Can you work these out from the drawing? Everything is in mm from the part's minimum corner. A direction names the side the tool comes from. Round coordinates to 2 decimals unless told otherwise and drop trailing zeros. Order: outer loops, then holes, each group sorted by start corner. A loop starts at its lowest first (then second) coordinate and runs counter-clockwise, first axis right, second up. Notation, with made-up numbers: (39.25, -34.5) -> (45.25, -34.5) arc R28 ccw to (45.25, 1.5) -> close; hole circle Ø8 at (67.5, -19.75). An arc over 180 degrees is marked (long way). One line per item, written item: value.
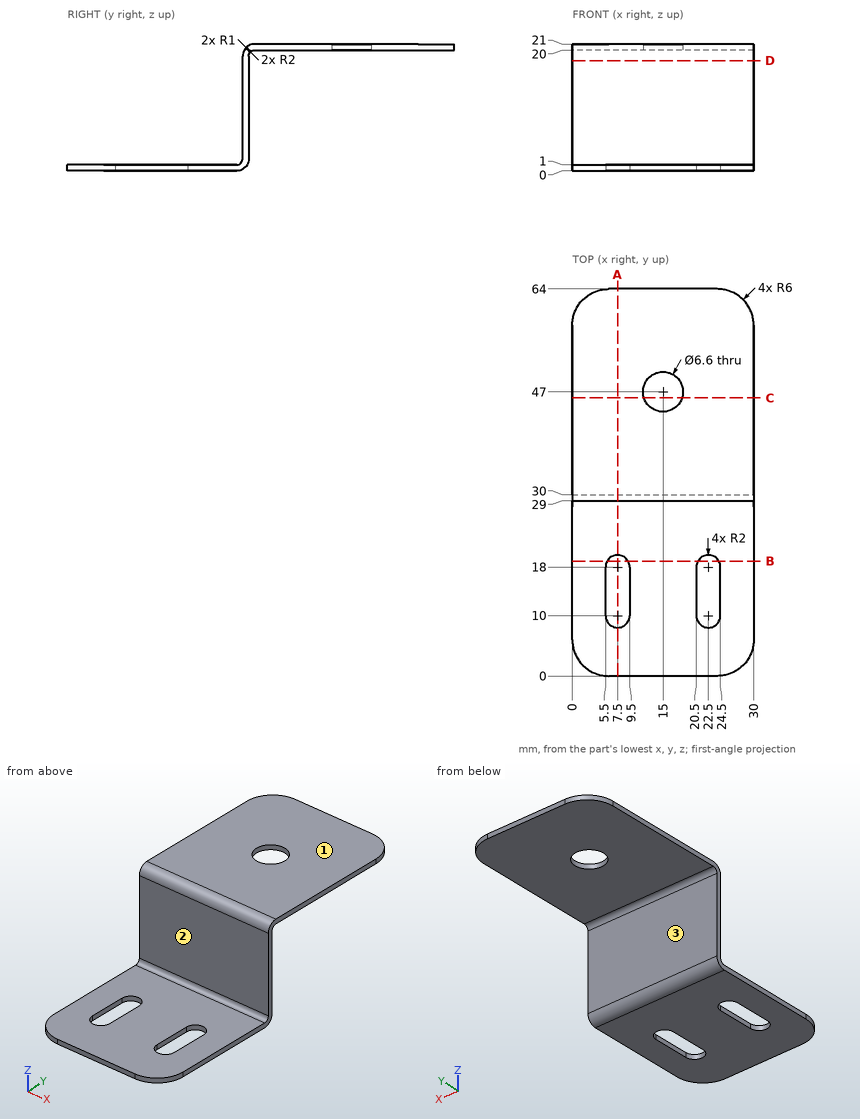
Q1. I want a section at C-C on y = 46. Write out the boundary of the cut face in (x, z).
Answers:
outline: (0, 20) -> (11.86, 20) -> (11.86, 21) -> (0, 21) -> close; (18.14, 20) -> (30, 20) -> (30, 21) -> (18.14, 21) -> close
Q2. I want a section at D-D on z = 18.25. Write out the boundary of the cut face in (x, y), then the cut area to 3 significant figures.
Answers:
outline: (0, 29) -> (30, 29) -> (30, 30) -> (0, 30) -> close
area: 30.0 mm2
Q3. I need wall thicknesses on line 1 along X through (y, z) = (47, 20.75); line 2 along Z through (x, y) = (8, 27); line 3 along Y through (x, z) = (24.5, 16.75). Which ranges of each line are inside material? Lowest first, please.
Answers:
line 1: 0 to 11.7, 18.3 to 30
line 2: 0 to 1
line 3: 29 to 30
Q4. For P1, Ø12, axis at x = 8.5, y = 48.5, coming from the -Z side; P2, Ø6, axis at x = 15, y = 47, coming from the +Z side; P3, Ø1.5, axis at x = 4, z = 9, coming from the +Y side, each with a flat end and sliding along its axis, tell me the tip position at first contact or that it passes through.
Answers:
P1: z = 20
P2: through
P3: y = 30
Q5. Which directions (+Z, -Z, +X, -X, +Y, -Y) give clear straight access to the entire face, cutting with the end or side of a thin tool? Please do the marked faces 1, 2 and 3.
Answers:
face 1: +Z, +X, -X, +Y, -Y
face 2: +Z, +X, -X, -Y
face 3: -Z, +X, -X, +Y
Q6. I want a section at B-B on y = 19. Write out the boundary of the cut face in (x, z), then the cut area to 3 significant figures.
Answers:
outline: (0, 0) -> (5.77, 0) -> (5.77, 1) -> (0, 1) -> close; (9.23, 0) -> (20.77, 0) -> (20.77, 1) -> (9.23, 1) -> close; (24.23, 0) -> (30, 0) -> (30, 1) -> (24.23, 1) -> close
area: 23.1 mm2
Q7. I want a section at A-A on x = 7.5. Write out the boundary of the cut face in (y, z).
Answers:
outline: (0, 0) -> (8, 0) -> (8, 1) -> (0, 1) -> close; (20, 0) -> (28, 0) arc R2 ccw to (30, 2) -> (30, 19) arc R1 cw to (31, 20) -> (64, 20) -> (64, 21) -> (31, 21) arc R2 ccw to (29, 19) -> (29, 2) arc R1 cw to (28, 1) -> (20, 1) -> close
